Autodesk Inventor part; units mm, degrees
ref_plane "YZ Plane" through (0, 0, 0) normal (1, 0, 0) x (0, 1, 0)
ref_plane "XZ Plane" through (0, 0, 0) normal (0, 1, 0) x (-1, 0, 0)
ref_plane "XY Plane" through (0, 0, 0) normal (0, 0, 1) x (1, 0, 0)
sketch "Sketch1" plane through (0, 0, 0) normal (1, 0, 0) x (0, 1, 0)
  line L0 (-9.1, 5) -> (9.1, 5)
  line L1 (9.1, 5) -> (9.1, -5)
  line L2 (9.1, -5) -> (-9.1, -5)
  line L3 (-9.1, -5) -> (-9.1, 5)
  line L4 (-9.1, 5) -> (9.1, -5) construction
  line L5 (9.1, 5) -> (-9.1, -5) construction
  point P0 (0, 0)
  dimension "d0" = 18.2
  dimension "d1" = 10
extrude "Extrusion1" add sketch "Sketch1" along normal blind 10
sketch "Sketch2" plane through (0, 9.1, 5) normal (0, 1, 0) x (1, 0, 0)
  line L0 (0, 5) -> (5, 5)
  circle A0 centre (5, 5) radius 2
  dimension "d4" = 5
  dimension "d5" = 4
extrude "Extrusion2" cut sketch "Sketch2" against normal blind 10
thread "Thread1"
properties part number "Rb PEEK - Soporte"
Read the model definition and answer for the solid it produces. Units are mm, in the model's axes. A direction names the side the tool comes from. Round coordinates to 2 decimals unless told otherwise and drop trailing zeros. Write each loop counter-clockwise with the first axis right and the second up, starting at its lowest first coordinate (ties: lowest second). Pieces come first, ordered by that corner, then holes. Notation, with made-up numbers: (29, 32) - (39, 32) arc R33 ccw to (39, 62) - close; hole circle Ø1 at (-17, -35.75). An arc over 180 degrees is marked (long way). Use CSV: the item, a comma, the result in double quotes.
Q1. Find section A-A, the plane x = 5. Write down the section's boundary in (y, z).
Values:
outline,"(-9.1, -5) - (9.1, -5) - (9.1, -2) - (-0.9, -2) - (-0.9, 2) - (9.1, 2) - (9.1, 5) - (-9.1, 5) - close"
Q2. Straight lines are drawn through the part: line 1 along Z through (x, y) = (5, 6.5); line 2 along Y through (x, z) = (6.25, 1.25); line 3 along Z through (x, y) = (4.5, 2). For each, find the intervals that lie inside material, in ascending order.
Values:
line 1,"z = -5 to -2, 2 to 5"
line 2,"y = -9.1 to -0.9"
line 3,"z = -5 to -1.94, 1.94 to 5"
Q3. Find section C-C, the plane z = 0. Write down the section's boundary in (x, y), then the cut area to 3 significant figures.
Values:
outline,"(0, -9.1) - (10, -9.1) - (10, 9.1) - (7, 9.1) - (7, -0.9) - (3, -0.9) - (3, 9.1) - (0, 9.1) - close"
area,"142 mm²"
Q4. Find section B-B, the plane y = 0. Write down the section's boundary in (x, z), then the cut area to 3 significant figures.
Values:
outline,"(0, -5) - (10, -5) - (10, 5) - (0, 5) - close; hole circle Ø4 at (5, 0)"
area,"87.4 mm²"
Q5. A tool of negligible diameter and unlimited length cuts with its end or side. For faces 4 (the flat face through (5, -0.9, 0)), 5 (the flat face through (5, 0, -5)), from which of +Z, -Z, +X, -X, +Y, -Y can it reach the whole face along a straight path? Write none if from no direction.
Values:
face 4,"+Y"
face 5,"-Z, +X, -X, +Y, -Y"
Q6. Determine the mould class of faces 1 (the cylindrical face through (3, 4, 0)), 2 (the flat face through (10, 0, 0)), 3 (the flat face through (5, -9.1, 0)) for opening direction X: +X half, -X half, draft (parallel to the pull), parting line (faces both ways), or undercut.
Values:
face 1,"undercut"
face 2,"+X half"
face 3,"draft"
Q7. This flat-tipped pin is pushed along its axis until it touches: pin 1 Ø3 at (x, z) = (5, 0) entering from +Y. Where does it stop, or does it pass through?
Values:
pin 1,"stops at y = -0.9"
